Work out the finished part from the listing and answer in its coordinate system (mm). A direction names the side the tool comes from. Give positions to 0.01 mm unless a question says otherwise; leave off trailing zeros. Loops run counter-clockwise (first coordinate to the right, second up) from the corner with the lowest first, then second, coordinate; pieces in that order, holes last. Notation, with made-up numbers: (56.5, -30) -> (96.5, -30) arc R22 cw to (96.5, 2) -> close; hole circle Ø7 at (19.25, -16.75). An arc over 180 degrees is marked (long way). Answer as CSV lines item,"result". Start each with the question number.
1. Find the intervals of material crossed by line 1 along X through (y, z) = (120, 0); line 2 along Y through (x, z) = (-5.5, 0); line 3 along Y through (x, z) = (-14, 41.5), in increasing order.
2. Find section C-C, the plane z = -7. Give the vertices of the cut face in (x, y).
3. Determine the mould class of faces 1 (the face through (-6.007, 35.496, 17.924)), 2 (the face through (-18.15, -30.42, -20.99)), 3 (the face through (0, -60, 18)) for opening direction Z: +Z half, -Z half, draft (parallel to the pull), parting line (faces both ways), or undercut.
4. A tool of negligible diameter and unlimited length cuts with its end or side. For faces 4 (the face through (-21, -30, 12)), 5 (the face through (0, 72, 37)), 6 (the face through (0, 62, 0)), 7 (the face through (3, -69.86, -9.54)), from which of +Z, -Z, +X, -X, +Y, -Y can it reach the whole face along a straight path? Write none if from no direction.
5. Find section B-B, the plane x = 5. Give the vertices of the cut face in (y, z).
6. Find section D-D, the plane y = 42.5. Give the vertices of the cut face in (x, z).
7. Find section A-A, the plane y = -37.5. Give the vertices of the cut face in (x, z).
8. Flat-ended cylindrical pins translate along their axes: pin 1 Ø5 at (x, y) = (-4.5, 101.5) entering from -Z; pin 2 Ø12.5 at (x, z) = (1, 29) entering from +Y; pin 3 Ø21 at (x, z) = (-1, 35.5) entering from -Y; pin 4 Ø8 at (y, z) = (-21, 40.5) entering from +X. Find the tip coordinate at first contact, or state that the pin passes through.
from build123d import *

# Parameters (mm, degrees)
SKETCH1_R      = 15.25
EXTRUDE1_DEPTH = 212
EXTRUDE2_DEPTH = 60
SKETCH3_R      = 20
EXTRUDE3_DEPTH = 72
SKETCH4_R      = 10
EXTRUDE4_DEPTH = 20
SKETCH5_R      = 4.1
EXTRUDE5_DEPTH = 15
SKETCH6_R      = 10
EXTRUDE6_DEPTH = 150
FILLET_1_R     = 10


with BuildPart() as part:
    # Sketch1 → Extrude1 (new body)
    with BuildSketch(Plane(origin=(0, 0, 0), x_dir=(1, 0, 0), z_dir=(0, 1, 0))):
        with Locations(Location((0, 0, 0), (0, 0, 270))):
            Circle(SKETCH1_R)
    extrude(amount=EXTRUDE1_DEPTH)

    # Sketch2 → Extrude2 (add)
    with BuildSketch(Plane.XZ):
        with BuildLine():
            Line((-1, 58), (1, 58))
            ThreePointArc((1, 58), (15.142135624, 52.142135624), (21, 38))
            Line((21, 38), (21, -24))
            Line((21, -24), (-21, -24))
            Line((-21, -24), (-21, 38))
            ThreePointArc((-21, 38), (-15.142135624, 52.142135624), (-1, 58))
        make_face()
    extrude(amount=EXTRUDE2_DEPTH)

    # Sketch3 → Extrude3 (add)
    with BuildSketch(Plane(origin=(0, 0, 0), x_dir=(1, 0, 0), z_dir=(0, 1, 0))):
        with Locations(Location((0, -37, 0), (0, 0, 90))):
            Circle(SKETCH3_R)
    extrude(amount=EXTRUDE3_DEPTH)

    # Sketch4 → Extrude4 (add)
    with BuildSketch(Plane.XZ.offset(60)):
        with Locations(Location((0, 0, 0), (0, 0, 270))):
            Circle(SKETCH4_R)
    extrude(amount=EXTRUDE4_DEPTH)

    # Sketch5 → Extrude5 (cut, symmetric)
    with BuildSketch(Plane(origin=(0, 0, 0), x_dir=(0, 0, -1), z_dir=(1, 0, 0))):
        with Locations((0, -72)):
            Circle(SKETCH5_R)
    extrude(amount=EXTRUDE5_DEPTH, both=True, mode=Mode.SUBTRACT)

    # Sketch6 → Extrude6 (cut)
    with BuildSketch(Plane(origin=(0, 212, 0), x_dir=(1, 0, 0), z_dir=(0, 1, 0))):
        with Locations(Location((0, 0, 0), (0, 0, 90))):
            Circle(SKETCH6_R)
    extrude(amount=-EXTRUDE6_DEPTH, mode=Mode.SUBTRACT)

    # Скругление1
    fillet_1_edges = [part.edges().sort_by_distance(p)[0] for p in [
        (21, -30, -24),
        (-21, -30, -24),
    ]]
    fillet(fillet_1_edges, radius=FILLET_1_R)


solid = part.part
Resolved:
1,line 1,"x = -15.25 to -10, 10 to 15.25"
1,line 2,"y = -80 to -76.1, -67.9 to 62"
1,line 3,"y = -60 to 72"
2,outline,"(-21, -60) -> (-7.14, -60) -> (-7.14, -80) -> (7.14, -80) -> (7.14, -60) -> (21, -60) -> (21, 0) -> (13.55, 0) -> (13.55, 212) -> (7.14, 212) -> (7.14, 62) -> (-7.14, 62) -> (-7.14, 212) -> (-13.55, 212) -> (-13.55, 0) -> (-21, 0) -> close"
3,face 1,"undercut"
3,face 2,"-Z half"
3,face 3,"draft"
4,face 4,"+Z, -Z, -X, +Y, -Y"
4,face 5,"+Z, +X, -X, +Y"
4,face 6,"+Y"
4,face 7,"-Y"
5,outline,"(-80, -8.66) -> (-60, -8.66) -> (-60, -24) -> (0, -24) -> (0, -14.41) -> (212, -14.41) -> (212, -8.66) -> (62, -8.66) -> (62, 8.66) -> (212, 8.66) -> (212, 14.41) -> (0, 14.41) -> (0, 17.64) -> (72, 17.64) -> (72, 56.36) -> (0, 56.36) -> (0, 57.6) -> (-60, 57.6) -> (-60, 8.66) -> (-80, 8.66) -> close; hole circle Ø8.2 at (-72, 0)"
6,outline,"circle Ø40 at (0, 37); circle Ø30.5 at (0, 0)"
7,outline,"(-21, -14) arc R10 ccw to (-11, -24) -> (11, -24) arc R10 ccw to (21, -14) -> (21, 38) arc R20 ccw to (1, 58) -> (-1, 58) arc R20 ccw to (-21, 38) -> close"
8,pin 1,"stops at z = -15.12"
8,pin 2,"stops at y = 72"
8,pin 3,"stops at y = -60"
8,pin 4,"stops at x = 21"
